Source: three-view drawing plus pictorial views. Frame: mm from the lowest corner of the part. A direction names the side the tool comes from. Round coordinates to 2 decimals unless told otherwise and drop trailing zeros. Loops run counter-clockwise (first coordinate to the right, second up) from the corner with the lowest first, then second, coordinate; pieces in that order, holes last. Notation, with made-up numbers: M 39,-33 L 92,-33 A27 ccw 92,-2 Z; hole C -27.75,10.5 d11. An arc over 180 degrees is marked long. Answer as a JSON object with one key per item and string values.
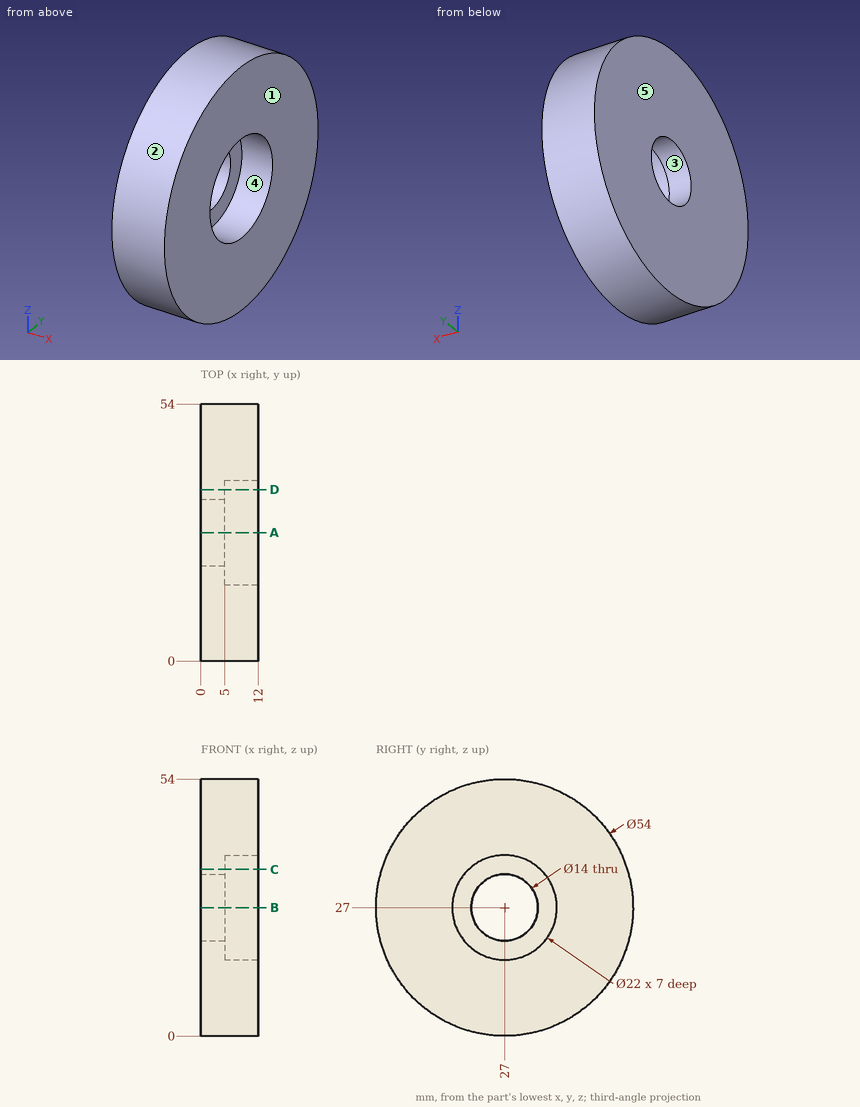
1) Line query: probe 1 along Y at (x, z) = (9.75, 27); probe 2 along X at (y, z) = (20, 32); probe 3 along Y at (x, z) = (11.25, 20.5). Output: solid intervals per line, ascending.
Geometry results:
{"probe 1": "0 to 16, 38 to 54", "probe 2": "0 to 5", "probe 3": "0.79 to 18.13, 35.87 to 53.21"}
2) Cut plane D-D on y = 36. Return the cut outline in (x, z).
Geometry results:
{"outline": "M 0,1.54 L 12,1.54 L 12,20.68 L 5,20.68 L 5,33.32 L 12,33.32 L 12,52.46 L 0,52.46 Z"}
3) Cut plane C-C on z = 35. Return the cut outline in (x, y).
Geometry results:
{"outline": "M 0,1.21 L 12,1.21 L 12,19.45 L 5,19.45 L 5,34.55 L 12,34.55 L 12,52.79 L 0,52.79 Z"}
4) Set-up query: the marked faces 4 and 5. Return all of +Z, -Z, +X, -X, +Y, -Y with unobstructed straight access to the full face (end or side cutting, diameter ignored); none if empty.
Geometry results:
{"face 4": "+X", "face 5": "+Z, -Z, -X, +Y, -Y"}
5) First-contact query: pin 1 (1.5 mm diameter, centred on x = 3.5, z = 11.5, fed in from -Y) (3 decimals); pin 2 (17.5 mm diameter, centred on y = 27, z = 27, fed in from +X); pin 3 (1.5 mm diameter, centred on x = 7.5, z = 19, fed in from -Y); pin 4 (12.5 mm diameter, centred on y = 27, z = 27, fed in from +X). Flat tips, straight axial feed; report the tip coordinate or a pass-through.
Geometry results:
{"pin 1": "y = 4.385", "pin 2": "x = 5", "pin 3": "y = 0.99", "pin 4": "through"}
6) Pull-direction query (Y, two-part tool) for the marked faces 1, 2 and 3; classes: +Y half, -Y half, draft (parallel to the pull), parting line (faces both ways), or undercut.
Geometry results:
{"face 1": "draft", "face 2": "parting line", "face 3": "undercut"}
7) Cut plane A-A on y = 27. Return the cut outline in (x, z), and give its area (3 significant figures).
Geometry results:
{"outline": "M 0,0 L 12,0 L 12,16 L 5,16 L 5,20 L 0,20 Z; M 0,34 L 5,34 L 5,38 L 12,38 L 12,54 L 0,54 Z", "area": "424 mm2"}
